```python
from build123d import *

# Parameters (mm, degrees)
SKETCH1_R           = 6.35
BOSS_EXTRUDE1_DEPTH = 6.35
CUT_EXTRUDE1_DEPTH  = 11.998522628


with BuildPart() as part:
    # Sketch1 → Boss-Extrude1 (new body)
    with BuildSketch(Plane(origin=(0, 0, 0), x_dir=(1, 0, 0), z_dir=(0, 1, 0))):
        with Locations(Location((0, 0, 0), (0, 0, 270))):
            Circle(SKETCH1_R)
    extrude(amount=-BOSS_EXTRUDE1_DEPTH)

    # Sketch2 → Cut-Extrude1 (cut, through all)
    with BuildSketch(Plane(origin=(0, 0, 0), x_dir=(1, 0, 0), z_dir=(0, 1, 0))):
        Polygon((2.2225, 3.84948292), (-2.2225, 3.84948292), (-4.445, 0), (-2.2225, -3.84948292), (2.2225, -3.84948292), (4.445, 0), align=None)
    extrude(amount=-CUT_EXTRUDE1_DEPTH, mode=Mode.SUBTRACT)


solid = part.part
```
Verification items for the finished model (mm, model axes). A direction names the side the tool comes from. Coordinates: 2 decimals unless noted, no trailing zeros. Write each loop counter-clockwise with the first axis right and the second up, starting at its lowest first coordinate (ties: lowest second). Pieces come first, ordered by that corner, then holes. Notation, with made-up numbers: M 54.5,89.5 L 61.5,89.5 A14 ccw 61.5,107.5 Z; hole C 10.5,-8.75 d4. An arc over 180 degrees is marked long. Answer as a JSON object with one key per item and string values. Group by question number.
(1) Cross-section at D-D, the plane z = 4.5. Record the cut outline in (x, y).
(2) Material ranges on line 1 (Z direction, x = 0.5, y = -2.75); line 2 (Z direction, x = 4.25, y = -3.5); line 3 (X direction, y = -1.25, z = -3), recorded low to high.
(3) Cross-section at C-C, the plane z = 3. Record the cut outline in (x, y), and give its area (3 significant figures).
(4) Cross-section at B-B, the plane x = 2.75. Record the cut outline in (y, z).
(5) Gauge pin test, flat ends, axial feed: pin 1 (3 mm diameter, centred on x = 4.5, y = -4, fed in from -Z); pin 2 (6 mm diameter, centred on x = 0, z = -0.5, fed in from +Y). Record the tip position at first contact, or that the pin passes through.
(6) Tool access check on faces 4 (the face through (3, -6.35, 3)), 5 (the face through (0, -3, 3.849)). Record the directions out of +Z, -Z, +X, -X, +Y, -Y that give a thin tool (end or side, any length) a straight path to the whole face; none if there is none.
(7) Release check for a two-part mould opening along X. For faces 1 (the face through (3.32, -3.13, 1.95)), 2 (the face through (-3.86, -3.13, -5.04)), 3 (the face through (3, 0, 3)) record: +X half, -X half, draft (parallel to the pull), parting line (faces both ways), or undercut.
Reply:
{
 "1": {"outline": "M -4.48,-6.35 L 4.48,-6.35 L 4.48,0 L -4.48,0 Z"},
 "2": {"line 1": "-6.33 to -3.85, 3.85 to 6.33", "line 2": "-4.72 to -0.34, 0.34 to 4.72", "line 3": "-5.6 to -2.71, 2.71 to 5.6"},
 "3": {"outline": "M -5.6,-6.35 L -2.71,-6.35 L -2.71,0 L -5.6,0 Z; M 2.71,-6.35 L 5.6,-6.35 L 5.6,0 L 2.71,0 Z", "area": "36.6 mm²"},
 "4": {"outline": "M -6.35,-5.72 L 0,-5.72 L 0,-2.94 L -6.35,-2.94 Z; M -6.35,2.94 L 0,2.94 L 0,5.72 L -6.35,5.72 Z"},
 "5": {"pin 1": "z = -5.6", "pin 2": "through"},
 "6": {"face 4": "+Z, -Z, +X, -X, -Y", "face 5": "+Y, -Y"},
 "7": {"face 1": "undercut", "face 2": "parting line", "face 3": "draft"}
}
